from build123d import *

# Parameters (mm, degrees)
F0_W     = 38.1
F0_H     = 25.4
F1_DEPTH = 25.4
F2_R     = 38.1
F3_DEPTH = 25.4
F4_DEPTH = 12.7
F5_DEPTH = 50.8
F7_DEPTH = 25.4


with BuildPart() as f1:
    # F0 (on Top) → F1 (new body)
    with BuildSketch(Plane.XY):
        with BuildLine():
            Line((0, 152.4), (0, 0))
            Line((0, 0), (203.2, 0))
            ThreePointArc((203.2, 0), (212.180256, 3.719744), (215.9, 12.7))
            Line((215.9, 12.7), (215.9, 38.1))
            ThreePointArc((215.9, 38.1), (219.619744, 47.080256), (228.6, 50.8))
            Line((228.6, 50.8), (254, 50.8))
            Line((254, 50.8), (254, 63.5))
            Line((254, 63.5), (228.6, 63.5))
            ThreePointArc((228.6, 63.5), (215.9, 76.2), (228.6, 88.9))
            Line((228.6, 88.9), (254, 88.9))
            Line((254, 88.9), (254, 101.6))
            Line((254, 101.6), (228.6, 101.6))
            ThreePointArc((228.6, 101.6), (219.619744, 105.319744), (215.9, 114.3))
            Line((215.9, 114.3), (215.9, 139.7))
            ThreePointArc((215.9, 139.7), (212.180256, 148.680256), (203.2, 152.4))
            Line((203.2, 152.4), (0, 152.4))
        make_face()
        with BuildLine():
            ThreePointArc((177.8, 50.8), (190.5, 38.1), (177.8, 25.4))
            Line((177.8, 25.4), (101.6, 25.4))
            ThreePointArc((101.6, 25.4), (88.9, 38.1), (101.6, 50.8))
            Line((101.6, 50.8), (177.8, 50.8))
        make_face(mode=Mode.SUBTRACT)
        with Locations((44.45, 76.2)):
            Rectangle(F0_W, F0_H, mode=Mode.SUBTRACT)
        with BuildLine():
            ThreePointArc((177.8, 127), (190.5, 114.3), (177.8, 101.6))
            Line((177.8, 101.6), (101.6, 101.6))
            ThreePointArc((101.6, 101.6), (88.9, 114.3), (101.6, 127))
            Line((101.6, 127), (177.8, 127))
        make_face(mode=Mode.SUBTRACT)
        with BuildLine():
            Line((228.6, 63.5), (254, 63.5))
            Line((254, 63.5), (254, 88.9))
            Line((254, 88.9), (228.6, 88.9))
            ThreePointArc((228.6, 88.9), (215.9, 76.2), (228.6, 63.5))
        make_face()
        with Locations((44.45, 76.2)):
            Rectangle(F0_W, F0_H)
    extrude(amount=-F1_DEPTH)

    # F2 (on face) → F3 (join)
    with BuildSketch(Plane(origin=(0, 0, 0), x_dir=(0, -1, 0), z_dir=(-1, 0, 0))):
        with BuildLine():
            Line((-152.4, 101.6), (-152.4, 0))
            Line((-152.4, 0), (0, 0))
            Line((0, 0), (0, 101.6))
            ThreePointArc((0, 101.6), (-76.2, 177.8), (-152.4, 101.6))
        make_face()
        with Locations((-76.2, 101.6)):
            Circle(F2_R, mode=Mode.SUBTRACT)
    extrude(amount=-F3_DEPTH)

    # F0 (on Top) → F4 (cut)
    with BuildSketch(Plane.XY):
        with BuildLine():
            Line((228.6, 63.5), (254, 63.5))
            Line((254, 63.5), (254, 88.9))
            Line((254, 88.9), (228.6, 88.9))
            ThreePointArc((228.6, 88.9), (215.9, 76.2), (228.6, 63.5))
        make_face()
    extrude(amount=-F4_DEPTH, mode=Mode.SUBTRACT)

    # F0 (on Top) → F5 (join)
    with BuildSketch(Plane.XY):
        with Locations((44.45, 76.2)):
            Rectangle(F0_W, F0_H)
    extrude(amount=F5_DEPTH)

    # F6 (on face) → F7 (cut)
    with BuildSketch(Plane.XZ.offset(-63.5)):
        Polygon((25.4, 50.8), (63.5, 0), (63.5, 50.8), align=None)
    extrude(amount=-F7_DEPTH, mode=Mode.SUBTRACT)


solid = f1.part
Part model, mm, in its own coordinate system. A direction names the side the tool comes from. Coordinates: 2 decimals unless noted, no trailing zeros. Order: outer loops, then holes, each group sorted by start corner. A loop starts at its lowest first (then second) coordinate and runs counter-clockwise, first axis right, second up.
(1) Slice it at C-C, the plane z = 88. Write the cut outline in (x, y).
Check sheet entries:
outline: (0, 0) - (25.4, 0) - (25.4, 40.61) - (0, 40.61) - close; (0, 111.79) - (25.4, 111.79) - (25.4, 152.4) - (0, 152.4) - close
(2) Pin check, flat tips, straight feed: pin 1 Ø1 at (y, z) = (56, 70.5) entering from +X; pin 2 Ø6 at (y, z) = (116, 126.5) entering from +X; pin 3 Ø4 at (x, z) = (235, -8.5) entering from +Y; pin 4 Ø7.5 at (x, z) = (238.5, -19) entering from -Y. Stop position of each tip, or through.
Check sheet entries:
pin 1: passes through
pin 2: stops at x = 25.4
pin 3: stops at y = 101.6
pin 4: stops at y = 50.8
(3) Probe L1, parallel to Z at x = 7, y = 76; L2, parallel to Y at x = 7, z = 101; L3, parallel to X at y = 107, z = 58.5. List the from-to ranges inside material, lowest first.
Check sheet entries:
L1: z = -25.4 to 63.5, 139.7 to 177.8
L2: y = 0 to 38.1, 114.3 to 152.4
L3: x = 0 to 25.4
(4) Pull direction Y, two halves, no side cores. Call faces 4 (the face through (219.52, 46.98, -12.52)), 5 (the face through (215.9, 127, -13)), 6 (the face through (190.497, 38.379, -12.522)): pulls with the +Y half, pulls with the -Y half, needs draft (parallel to the pull), parting line crosses it, or undercut.
Check sheet entries:
face 4: pulls with the -Y half
face 5: needs draft
face 6: undercut
(5) Slice it at D-D, the plane y = 47. Write the cut outline in (x, z).
Check sheet entries:
outline: (0, -25.4) - (92.54, -25.4) - (92.54, 0) - (25.4, 0) - (25.4, 77.13) - (0, 77.13) - close; (0, 126.07) - (25.4, 126.07) - (25.4, 171.98) - (0, 171.98) - close; (186.86, -25.4) - (219.54, -25.4) - (219.54, 0) - (186.86, 0) - close
(6) Tool access for faces 1 (the face through (138, 77, 0)), 2 (the face through (215.9, 25, -13)), 3 (the face through (139, 50.8, -13)): list every direction of +Z, -Z, +X, -X, +Y, -Y with a clear straight run to the whole face (end or side of a thin tool).
Check sheet entries:
face 1: +Z, +X
face 2: +Z, -Z, +X, -Y
face 3: +Z, -Z
(7) Slice it at A-A, the plane x = 121.5. Write the cut outline in (y, z), and give its area (3 significant figures).
Check sheet entries:
outline: (0, -25.4) - (25.4, -25.4) - (25.4, 0) - (0, 0) - close; (50.8, -25.4) - (101.6, -25.4) - (101.6, 0) - (50.8, 0) - close; (127, -25.4) - (152.4, -25.4) - (152.4, 0) - (127, 0) - close
area: 2,580 mm2
(8) Slice it at B-B, the plane y = 76.2. Write the cut outline in (x, z).
Check sheet entries:
outline: (0, -25.4) - (254, -25.4) - (254, -12.7) - (215.9, -12.7) - (215.9, 0) - (63.5, 0) - (25.4, 50.8) - (25.4, 63.5) - (0, 63.5) - close; (0, 139.7) - (25.4, 139.7) - (25.4, 177.8) - (0, 177.8) - close
